Source: CAD feature listing. Evaluate the final solid. Frame: model axes, mm. Face numbers are marked on the shaded views. A direction names the side the tool comes from. Coordinates: 2 decimals unless noted, no trailing zeros. Loops run counter-clockwise (first coordinate to the right, second up) from the corner with the lowest first, then second, coordinate; pieces in that order, holes last.
Item 1: Section query B-B, the plane y = 20. Return the cut outline in (x, z).
Item 2: Section query A-A, the plane x = 18. Return the cut outline in (y, z) (3 decimals), then the cut area to 3 significant figures.
Item 3: Pin query (flat end, axial travel): pin 1 Ø0.5 at (y, z) = (4.5, 67.5) entering from -X (3 decimals); pin 2 Ø12 at (x, y) = (-15.5, 21) entering from +Z; pin 3 Ø0.8 at (y, z) = (4.5, -67.5) entering from -X (3 decimals); pin 4 Ø8 at (x, z) = (-33.5, 32.5) entering from -Y. Return the tip coordinate at first contact, or that it passes through.
Item 4: Line query: probe 1 along Z at (x, y) = (3, 14); probe 2 along Y at (x, z) = (-9, 65) (3 decimals); probe 3 along Z at (x, y) = (39, 26.5). Output: solid intervals per line, ascending.
Item 5: Reachability of the marked faces 1, 2 and 3 from +Z, -Z, +X, -X, +Y, -Y: full face, straight path, thin tool, end or side. Return the list, or none.
Item 6: Section query D-D, the plane y = 4. State how many separate pieces and enclosed holes the cut face has, then the cut area to 3 significant figures.
Item 7: Section query C-C, the plane z = -61. Return the cut outline in (x, y) (3 decimals), then the cut area to 3 significant figures.
Autodesk Inventor part; units mm, degrees
ref_plane "YZ Plane" through (0, 0, 0) normal (1, 0, 0) x (0, 1, 0)
ref_plane "XZ Plane" through (0, 0, 0) normal (0, 1, 0) x (-1, 0, 0)
ref_plane "XY Plane" through (0, 0, 0) normal (0, 0, 1) x (1, 0, 0)
sketch "Sketch1" plane through (0, 0, 0) normal (0, 1, 0) x (-1, 0, 0)
  line L0 (-44.45, 73.025) -> (44.45, 73.025)
  line L1 (44.45, 73.025) -> (44.45, -73.025)
  line L2 (44.45, -73.025) -> (-44.45, -73.025)
  line L3 (-44.45, -73.025) -> (-44.45, 73.025)
  line L4 (-44.45, 73.025) -> (44.45, -73.025) construction
  line L5 (44.45, 73.025) -> (-44.45, -73.025) construction
  point P0 (0, 0)
  dimension "d0" = 88.9
  dimension "d1" = 146.05
extrude "Extrusion1" add sketch "Sketch1" along normal blind 9.525
sketch "Sketch2" plane through (0, 9.525, 0) normal (0, 1, 0) x (1, 0, 0)
  line L0 (44.45, -57.15) -> (-44.45, -57.15)
  line L1 (-44.45, -57.15) -> (-44.45, 57.15)
  line L2 (-44.45, 57.15) -> (44.45, 57.15)
  line L3 (44.45, 57.15) -> (44.45, -57.15)
  line L4 (44.45, -57.15) -> (-44.45, 57.15) construction
  line L5 (-44.45, -57.15) -> (44.45, 57.15) construction
  point P0 (0, 0)
  dimension "d4" = 88.9
  dimension "d5" = 114.3
extrude "Extrusion2" add sketch "Sketch2" along normal blind 30
sketch "Sketch3" plane through (0, 0, 0) normal (0, -1, 0) x (1, 0, 0)
  line L0 (-37.5007, -70.0145) -> (-27.5007, -70.0145)
  line L1 (-27.5007, -70.0145) -> (-27.5007, -65.0145)
  line L2 (-27.5007, -65.0145) -> (-37.5007, -65.0145)
  line L3 (-37.5007, -65.0145) -> (-37.5007, -70.0145)
  line L4 (-37.5007, -70.0145) -> (-27.5007, -65.0145) construction
  line L5 (-27.5007, -70.0145) -> (-37.5007, -65.0145) construction
  line L6 (-37.5007, 64.9855) -> (-27.5007, 64.9855)
  line L7 (-27.5007, 64.9855) -> (-27.5007, 69.9855)
  line L8 (-27.5007, 69.9855) -> (-37.5007, 69.9855)
  line L9 (-37.5007, 69.9855) -> (-37.5007, 64.9855)
  line L10 (-37.5007, 64.9855) -> (-27.5007, 69.9855) construction
  line L11 (-27.5007, 64.9855) -> (-37.5007, 69.9855) construction
  line L12 (-44.45, -73.025) -> (44.45, -73.025)
  line L13 (27.4993, -70.0145) -> (37.4993, -70.0145)
  line L14 (37.4993, -70.0145) -> (37.4993, -65.0145)
  line L15 (37.4993, -65.0145) -> (27.4993, -65.0145)
  line L16 (27.4993, -65.0145) -> (27.4993, -70.0145)
  line L17 (27.4993, -70.0145) -> (37.4993, -65.0145) construction
  line L18 (37.4993, -70.0145) -> (27.4993, -65.0145) construction
  line L19 (44.45, -73.025) -> (44.45, 73.025)
  line L20 (37.4993, 69.9855) -> (27.4993, 69.9855)
  line L21 (27.4993, 69.9855) -> (27.4993, 64.9855)
  line L22 (27.4993, 64.9855) -> (37.4993, 64.9855)
  line L23 (37.4993, 64.9855) -> (37.4993, 69.9855)
  line L24 (37.4993, 69.9855) -> (27.4993, 64.9855) construction
  line L25 (27.4993, 69.9855) -> (37.4993, 64.9855) construction
  point P0 (0, 0)
  point P1 (-32.5007, -67.5145)
  point P2 (-32.5007, 67.4855)
  point P3 (32.4993, -67.5145)
  point P4 (-42.8625, -71.4375)
  point P5 (32.4993, 67.4855)
  dimension "d8" = 10
  dimension "d9" = 5
  dimension "d10" = 10
  dimension "d11" = 5
  dimension "d12" = 0
  dimension "d13" = 135
  dimension "d14" = 5.5105
  dimension "d15" = 10
  dimension "d16" = 5
  dimension "d17" = 65
  dimension "d18" = 5.5105
  dimension "d19" = 11.9507
  dimension "d20" = 5
  dimension "d21" = 10
  dimension "d22" = 135
  dimension "d23" = 11.9507
extrude "Extrusion3" cut sketch "Sketch3" against normal blind 30
fillet "Fillet1" radius 2.159 16 edges at (-27.5007, 4.7625, 64.9855) (-27.5007, 4.7625, 69.9855) (-37.5007, 4.7625, 69.9855) (-37.5007, 4.7625, 64.9855) (37.4993, 4.7625, 64.9855) (37.4993, 4.7625, 69.9855) (27.4993, 4.7625, 64.9855) (27.4993, 4.7625, 69.9855) (27.4993, 4.7625, -65.0145) (37.4993, 4.7625, -70.0145) (37.4993, 4.7625, -65.0145) (27.4993, 4.7625, -70.0145) (-27.5007, 4.7625, -65.0145) (-27.5007, 4.7625, -70.0145) (-37.5007, 4.7625, -65.0145) (-37.5007, 4.7625, -70.0145)
fillet "Fillet2" radius 6.35 1 edges at (-44.45, 24.525, -57.15)
fillet "Fillet3" radius 6.35 8 edges at (-44.45, 24.525, 57.15) (44.45, 24.525, 57.15) (44.45, 24.525, -57.15) (-42.5901, 39.525, -55.2901) (-44.45, 39.525, 3.175) (3.175, 39.525, -57.15) (44.45, 39.525, 0) (0, 39.525, 57.15)
chamfer "Chamfer1" distance 8.89 angle 45 4 edges at (44.45, 4.7625, 73.025) (-44.45, 4.7625, 73.025) (44.45, 4.7625, -73.025) (-44.45, 4.7625, -73.025)
equation "\"d20\" = d11"
equation "\"d21\" = d10"
properties part number "24v Converter"
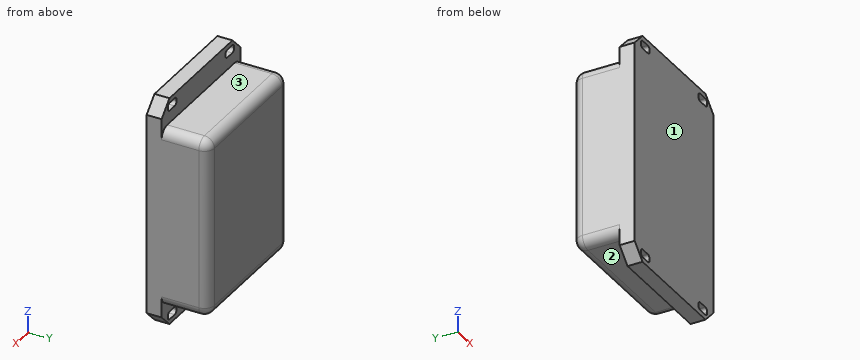
Verdict:
1. outline: (-44.45, -50.8) arc R6.35 ccw to (-38.1, -57.15) - (38.1, -57.15) arc R6.35 ccw to (44.45, -50.8) - (44.45, 50.8) arc R6.35 ccw to (38.1, 57.15) - (-38.1, 57.15) arc R6.35 ccw to (-44.45, 50.8) - close
2. outline: (0, -73.025) - (9.525, -73.025) - (9.525, -57.15) - (33.175, -57.15) arc R6.35 ccw to (39.525, -50.8) - (39.525, 50.8) arc R6.35 ccw to (33.175, 57.15) - (9.525, 57.15) - (9.525, 73.025) - (0, 73.025) - close
2. area: 4,800 mm2
3. pin 1: stops at x = -41.335
3. pin 2: stops at z = 57.15
3. pin 3: stops at x = -41.485
3. pin 4: stops at y = 0
4. probe 1: z = -57.15 to 57.15
4. probe 2: y = 0 to 9.525
4. probe 3: z = -57.09 to 57.09
5. face 1: +Z, -Z, +X, -X, -Y
5. face 2: -Z, +X, -X, +Y
5. face 3: +Z, +X, -X, +Y
6. separate pieces: 1
6. enclosed holes: 4
6. area: 12,600 mm2
7. outline: (-44.45, 0) - (44.45, 0) - (44.45, 9.525) - (-44.45, 9.525) - close
7. area: 847 mm2
